Model file for the job. Use its own axes, mm. Give positions to 0.01 mm unless a question says otherwise; leave off trailing zeros. Order: outer loops, then holes, each group sorted by start corner. A loop starts at its lowest first (then second) coordinate and runs counter-clockwise, first axis right, second up. Notation, with made-up numbers: (23.5, -35) - (45.5, -35) arc R15 cw to (45.5, -24) - close; hole circle Ø8 at (3, 8.25). An arc over 180 degrees is marked (long way). Return JSON: item names as keys, results as strings. Group by question number.
from build123d import *

# Parameters (mm, degrees)
BOSS_EXTRUDE1_DEPTH = 1.5875
CUT_EXTRUDE1_DEPTH  = 3.175
FILLET1_R           = 8.89
SKETCH3_W           = 234.443386257
SKETCH3_H           = 422.563019086
CUT_EXTRUDE2_DEPTH  = 134.35
CUT_EXTRUDE3_DEPTH  = 4.175


with BuildPart() as part:
    # Sketch1 → Boss-Extrude1 (new body, symmetric)
    with BuildSketch(Plane.XY):
        with BuildLine():
            Line((-120.187952283, -34.272453), (-93.24718392, -61.213221363))
            Line((-93.24718392, -61.213221363), (-94.292689271, -70.797689271))
            ThreePointArc((-94.292689271, -70.797689271), (-77.124658044, -85.289234251), (-57.767453, -96.692952283))
            ThreePointArc((-57.767453, -96.692952283), (94.292689271, 117.787689271), (-120.187952283, -34.272453))
        make_face()
    extrude(amount=BOSS_EXTRUDE1_DEPTH, both=True)

    # Sketch2 → Cut-Extrude1 (cut)
    with BuildSketch(Plane.XY.offset(1.5875)):
        with BuildLine():
            Line((-77.304798152, -55.60299244), (-78.320318415, -64.912577861))
            ThreePointArc((-78.320318415, -64.912577861), (94.997930523, 93.675946819), (-107.51910025, -25.388690342))
            Line((-107.51910025, -25.388690342), (-77.304798152, -55.60299244))
        make_face()
    extrude(amount=-CUT_EXTRUDE1_DEPTH, mode=Mode.SUBTRACT)

    # Fillet1
    fillet1_edges = [part.edges().sort_by_distance(p)[0] for p in [
        (-77.304798152, -55.60299244, 0),
        (-107.51910025, -25.388690342, 0),
        (-78.320318415, -64.912577861, 0),
        (-93.24718392, -61.213221363, -0.79375),
        (-120.187952283, -34.272453, -0.79375),
        (-94.292689271, -70.797689271, -0.79375),
    ]]
    fillet(fillet1_edges, radius=FILLET1_R)

    # Sketch3 → Cut-Extrude2 (cut, through all)
    with BuildSketch(Plane(origin=(0, 0, 0), x_dir=(0, 0, -1), z_dir=(1, 0, 0))):
        with Locations((10.168628802, 16.433452221)):
            Rectangle(SKETCH3_W, SKETCH3_H)
    extrude(amount=-CUT_EXTRUDE2_DEPTH, mode=Mode.SUBTRACT)

    # Sketch4 → Cut-Extrude3 (cut, through all)
    with BuildSketch(Plane(origin=(0, 0, -1.5875), x_dir=(-1, 0, 0), z_dir=(0, 0, -1))):
        with BuildLine():
            Line((-3.302, 156.804111827), (-3.302, 147.955))
            Line((-3.302, 147.955), (0, 147.955))
            Line((0, 147.955), (0, 156.845))
            ThreePointArc((0, 156.845), (-1.651126573, 156.834777565), (-3.302, 156.804111827))
        make_face()
        with BuildLine():
            Line((-105.489605782, 89.621888205), (-113.138876948, 94.076987949))
            ThreePointArc((-113.138876948, 94.076987949), (-114.023976238, 92.638006465), (-114.890774539, 91.187927443))
            Line((-114.890774539, 91.187927443), (-107.18979641, 86.702712453))
            Line((-107.18979641, 86.702712453), (-105.489605782, 89.621888205))
        make_face()
        with BuildLine():
            Line((-109.566752285, -35.631551273), (-117.216023462, -40.086650998))
            ThreePointArc((-117.216023462, -40.086650998), (-116.401122895, -41.566517726), (-115.567539805, -43.035942))
            Line((-115.567539805, -43.035942), (-107.866561664, -38.550727029))
            Line((-107.866561664, -38.550727029), (-109.566752285, -35.631551273))
        make_face()
        with BuildLine():
            Line((-3.302, -100.965), (-3.302, -109.814111827))
            ThreePointArc((-3.302, -109.814111827), (-1.651126573, -109.844777565), (0, -109.855))
            Line((0, -109.855), (0, -100.965))
            Line((0, -100.965), (-3.302, -100.965))
        make_face()
    extrude(amount=-CUT_EXTRUDE3_DEPTH, mode=Mode.SUBTRACT)


solid = part.part
(1) Slice it at C-C (x = 80). Give the cut face in (y, z), and give its area (3 significant figures).
(2) Slice it at B-B (z = 0.65). Give the cut face in (x, y) (3 decimals).
(3) Slice it at A-A (x = 61). Give the cut face in (y, z).
(4) Pull direction X, two halves, no side cores. Call faces 1 (the face through (111.094, 88.977, -0.022)), 2 (the face through (116, -6, -1.588)), 3 (the face through (111.771, -40.825, -0.022)), 4 (the face through (67.348, -91.598, 0.022)): released by +X, released by -X, zero draft, split by the parting line, or undercut.
(5) Drop flat-ended pins along their axis: pin 1 Ø1 at (x, z) = (117.5, 0.5) entering from +Y; pin 2 Ø1.6 at (y, z) = (-106, 0) entering from -X. Give the stop position or say it passes through.
(6) Slice it at D-D (y = 114). Give the cut face in (x, z), and give its area (3 significant figures).
(7) Drill centre lines: L1, parallel to Y at x = 109, z = -1.4; L2, parallel to Y at x = 15.5, z = 1.4; L3, parallel to Y at x = 54.5, z = 0.7. Where is each one in solid material? Low to high.
Result set:
{
 "1": {"outline": "(-83.19, -1.59) - (-63.4, -1.59) - (-63.4, 1.59) - (-83.19, 1.59) - close; (110.39, -1.59) - (130.18, -1.59) - (130.18, 1.59) - (110.39, 1.59) - close", "area": "126 mm²"},
 "2": {"outline": "(0, -100.965) - (3.302, -100.965) - (3.302, -109.814) arc R133.35 ccw to (115.568, -43.036) - (107.867, -38.551) - (109.567, -35.632) - (117.216, -40.087) arc R133.35 ccw to (114.891, 91.188) - (107.19, 86.703) - (105.49, 89.622) - (113.139, 94.077) arc R133.35 ccw to (3.302, 156.804) - (3.302, 147.955) - (0, 147.955) - (0, 141.605) arc R118.11 cw to (0, -94.615) - close"},
 "3": {"outline": "(-95.09, -1.59) - (-77.64, -1.59) - (-77.64, 1.59) - (-95.09, 1.59) - close; (124.63, -1.59) - (142.08, -1.59) - (142.08, 1.59) - (124.63, 1.59) - close"},
 "4": {"face 1": "undercut", "face 2": "zero draft", "face 3": "undercut", "face 4": "released by +X"},
 "5": {"pin 1": "stops at y = 87.47", "pin 2": "stops at x = 3.3"},
 "6": {"outline": "(75.89, -1.59) - (97.93, -1.59) - (97.93, 1.59) - (75.89, 1.59) - close", "area": "70.0 mm²"},
 "7": {"L1": "y = -53.32 to -39.21, -36.6 to -21.99, 68.98 to 87.76, 91.67 to 100.31", "L2": "y = -108.95 to -93.59, 140.58 to 155.94", "L3": "y = -98.21 to -81.29, 128.28 to 145.2"}
}
